Work out the finished part from the listing and answer in its coordinate system (mm). Round coordinates to 2 decimals unless told otherwise and drop trailing zeros. Write each loop counter-clockwise with the first axis right and the second up, starting at its lowest first coordinate (ties: lowest second). Pieces come first, ordered by that corner, then holes. Notation, with made-up numbers: (54.25, 24.5) -> (77.25, 24.5) arc R6 cw to (77.25, 29.5) -> close; hole circle Ø9 at (66.5, -12). An arc over 180 degrees is marked (long way). One line per item, written item: value.
```python
from build123d import *

# Parameters (mm, degrees)
ESQUISSE1_R             = 2.75
ESQUISSE1_R_2           = 2.6
ESQUISSE1_R_3           = 2.1
ESQUISSE1_W             = 40.6
ESQUISSE1_H             = 3.4
ESQUISSE1_W_2           = 10
ESQUISSE1_H_2           = 15
BOSS_EXTRU_1_DEPTH      = 3
ENL_V_MAT_EXTRU_1_REACH = 5
ESQUISSE2_W             = 35
ESQUISSE2_H             = 8.195


with BuildPart() as part:
    # Esquisse1 → Boss.-Extru.1 (new body)
    with BuildSketch(Plane(origin=(0, 0, 0), x_dir=(-1, 0, 0), z_dir=(0, 0, -1))):
        Polygon((-14, 66), (-241, 66), (-241, 86), (-255, 86), (-255, 20), (-255, 0), (-241, 0), (-241, 20), (-14, 20), (-14, 0), (0, 0), (0, 86), (-14, 86), align=None)
        with Locations((-7, 81)):
            Circle(ESQUISSE1_R, mode=Mode.SUBTRACT)
        with Locations((-32, 43)):
            Circle(ESQUISSE1_R_2, mode=Mode.SUBTRACT)
        with Locations((-40, 43)):
            Circle(ESQUISSE1_R_2, mode=Mode.SUBTRACT)
        with Locations((-137.5, 39)):
            Circle(ESQUISSE1_R, mode=Mode.SUBTRACT)
        with Locations((-117.5, 39)):
            Circle(ESQUISSE1_R, mode=Mode.SUBTRACT)
        with Locations((-137.5, 59)):
            Circle(ESQUISSE1_R, mode=Mode.SUBTRACT)
        with Locations((-117.5, 59)):
            Circle(ESQUISSE1_R, mode=Mode.SUBTRACT)
        with Locations((-94.5, 51.805)):
            Circle(ESQUISSE1_R_3, mode=Mode.SUBTRACT)
        with Locations((-248, 37)):
            Circle(ESQUISSE1_R, mode=Mode.SUBTRACT)
        with Locations((-248, 5)):
            Circle(ESQUISSE1_R, mode=Mode.SUBTRACT)
        with Locations((-248, 49.000000164)):
            Circle(ESQUISSE1_R, mode=Mode.SUBTRACT)
        with Locations((-117.5, 49)):
            Circle(ESQUISSE1_R, mode=Mode.SUBTRACT)
        with Locations((-137.5, 49)):
            Circle(ESQUISSE1_R, mode=Mode.SUBTRACT)
        with Locations((-160.5, 51.805)):
            Circle(ESQUISSE1_R_3, mode=Mode.SUBTRACT)
        with Locations((-94.5, 34.195)):
            Circle(ESQUISSE1_R_3, mode=Mode.SUBTRACT)
        with Locations((-70.5, 34.195)):
            Circle(ESQUISSE1_R_3, mode=Mode.SUBTRACT)
        with Locations((-70.5, 51.805)):
            Circle(ESQUISSE1_R_3, mode=Mode.SUBTRACT)
        with Locations((-184.5, 34.195)):
            Circle(ESQUISSE1_R_3, mode=Mode.SUBTRACT)
        with Locations((-7, 37)):
            Circle(ESQUISSE1_R, mode=Mode.SUBTRACT)
        with Locations((-248, 81)):
            Circle(ESQUISSE1_R, mode=Mode.SUBTRACT)
        with Locations((-24, 43)):
            Circle(ESQUISSE1_R_2, mode=Mode.SUBTRACT)
        with Locations((-184.5, 51.805)):
            Circle(ESQUISSE1_R_3, mode=Mode.SUBTRACT)
        with Locations((-7, 5)):
            Circle(ESQUISSE1_R, mode=Mode.SUBTRACT)
        with Locations((-7, 49.000000164)):
            Circle(ESQUISSE1_R, mode=Mode.SUBTRACT)
        with Locations((-160.5, 34.195)):
            Circle(ESQUISSE1_R_3, mode=Mode.SUBTRACT)
        with Locations((-217.7, 58.5)):
            Rectangle(ESQUISSE1_W, ESQUISSE1_H, mode=Mode.SUBTRACT)
        with BuildLine():
            Line((-214.7, 31.8), (-220.7, 31.8))
            ThreePointArc((-220.7, 31.8), (-231.9, 43), (-220.7, 54.2))
            Line((-220.7, 54.2), (-214.7, 54.2))
            ThreePointArc((-214.7, 54.2), (-203.5, 43), (-214.7, 31.8))
        make_face(mode=Mode.SUBTRACT)
        with Locations((-217.7, 27.5)):
            Rectangle(ESQUISSE1_W, ESQUISSE1_H, mode=Mode.SUBTRACT)
        with Locations((-52, 43)):
            Rectangle(ESQUISSE1_W_2, ESQUISSE1_H_2, mode=Mode.SUBTRACT)
    extrude(amount=-BOSS_EXTRU_1_DEPTH)

    # Esquisse2 → Enlèv. mat.-Extru.1 (cut, up to next)
    with BuildSketch(Plane.XY.offset(3), mode=Mode.PRIVATE) as enl_v_mat_extru_1_sk1:
        with Locations((82.5, 61.9025)):
            Rectangle(ESQUISSE2_W, ESQUISSE2_H)
    enl_v_mat_extru_1_tool1 = extrude(enl_v_mat_extru_1_sk1.sketch, amount=-ENL_V_MAT_EXTRU_1_REACH, mode=Mode.PRIVATE) & part.part
    add(enl_v_mat_extru_1_tool1.solids().sort_by_distance((82.5, 61.9025, 3))[0], mode=Mode.SUBTRACT)
    # Esquisse2 → Enlèv. mat.-Extru.1 (cut, up to next)
    with BuildSketch(Plane.XY.offset(3), mode=Mode.PRIVATE) as enl_v_mat_extru_1_sk2:
        with Locations((82.5, 24.0975)):
            Rectangle(ESQUISSE2_W, ESQUISSE2_H)
    enl_v_mat_extru_1_tool2 = extrude(enl_v_mat_extru_1_sk2.sketch, amount=-ENL_V_MAT_EXTRU_1_REACH, mode=Mode.PRIVATE) & part.part
    add(enl_v_mat_extru_1_tool2.solids().sort_by_distance((82.5, 24.0975, 3))[0], mode=Mode.SUBTRACT)
    # Esquisse2 → Enlèv. mat.-Extru.1 (cut, up to next)
    with BuildSketch(Plane.XY.offset(3), mode=Mode.PRIVATE) as enl_v_mat_extru_1_sk3:
        with Locations((172.5, 24.0975)):
            Rectangle(ESQUISSE2_W, ESQUISSE2_H)
    enl_v_mat_extru_1_tool3 = extrude(enl_v_mat_extru_1_sk3.sketch, amount=-ENL_V_MAT_EXTRU_1_REACH, mode=Mode.PRIVATE) & part.part
    add(enl_v_mat_extru_1_tool3.solids().sort_by_distance((172.5, 24.0975, 3))[0], mode=Mode.SUBTRACT)
    # Esquisse2 → Enlèv. mat.-Extru.1 (cut, up to next)
    with BuildSketch(Plane.XY.offset(3), mode=Mode.PRIVATE) as enl_v_mat_extru_1_sk4:
        with Locations((172.5, 61.9025)):
            Rectangle(ESQUISSE2_W, ESQUISSE2_H)
    enl_v_mat_extru_1_tool4 = extrude(enl_v_mat_extru_1_sk4.sketch, amount=-ENL_V_MAT_EXTRU_1_REACH, mode=Mode.PRIVATE) & part.part
    add(enl_v_mat_extru_1_tool4.solids().sort_by_distance((172.5, 61.9025, 3))[0], mode=Mode.SUBTRACT)


solid = part.part
```
(1) Find section B-B on x = 137.5. Give the vertices of the cut face in (y, z).
Reported:
outline: (20, 0) -> (36.25, 0) -> (36.25, 3) -> (20, 3) -> close; (41.75, 0) -> (46.25, 0) -> (46.25, 3) -> (41.75, 3) -> close; (51.75, 0) -> (56.25, 0) -> (56.25, 3) -> (51.75, 3) -> close; (61.75, 0) -> (66, 0) -> (66, 3) -> (61.75, 3) -> close
(2) Flat-ended cylindrical pins translate along their axes: pin 1 Ø5 at (x, y) = (7, 49) entering from +Z; pin 2 Ø1 at (x, z) = (154, 2) entering from +Y; pin 3 Ø0.9 at (x, z) = (179.5, 1) entering from +Y (3 decimals). Find the tip coordinate at first contact, or state that the pin passes through.
Reported:
pin 1: passes through
pin 2: stops at y = 66
pin 3: stops at y = 57.805
(3) Find section C-C on z = 1.95. Give the number of separate pieces and of enclosed holes in the cut face, plus the area to 3 significant figures.
Reported:
separate pieces: 1
enclosed holes: 29
area: 10,200 mm2
(4) Consider probe 1 along Y at (x, z) = (184.5, 0.9) (3 decimals); probe 2 along Y at (x, z) = (7, 0.75); probe 3 along X at (y, z) = (22, 1.15). Determine where each line is inside the solid, lowest interval first.
Reported:
probe 1: y = 28.195 to 32.095, 36.295 to 49.705, 53.905 to 57.805
probe 2: y = 0 to 2.25, 7.75 to 34.25, 39.75 to 46.25, 51.75 to 78.25, 83.75 to 86
probe 3: x = 0 to 65, 100 to 155, 190 to 255
(5) Find section A-A on x = 7. Give the vertices of the cut face in (y, z).
Reported:
outline: (0, 0) -> (2.25, 0) -> (2.25, 3) -> (0, 3) -> close; (7.75, 0) -> (34.25, 0) -> (34.25, 3) -> (7.75, 3) -> close; (39.75, 0) -> (46.25, 0) -> (46.25, 3) -> (39.75, 3) -> close; (51.75, 0) -> (78.25, 0) -> (78.25, 3) -> (51.75, 3) -> close; (83.75, 0) -> (86, 0) -> (86, 3) -> (83.75, 3) -> close
(6) Find section D-D on x = 61. Give the vertices of the cut face in (y, z), plus the area to 3 significant figures.
Reported:
outline: (20, 0) -> (66, 0) -> (66, 3) -> (20, 3) -> close
area: 138 mm2
(7) For a pull along X with two mould halves and no side action, classify faces 1 (the face through (129, 44, 3)), 2 (the face through (231.9, 42.8, 1.5)), 3 (the face through (42.063, 41.418, 1.479)) as pulls with the +X half, pulls with the -X half, needs draft (parallel to the pull), parting line crosses it, or undercut.
Reported:
face 1: needs draft
face 2: undercut
face 3: undercut
